Input: part model. Units: mm. Frame: model coordinates. A direction names the side the tool comes from. Give positions to 0.01 mm unless a question says otherwise; leave off trailing zeros. Loops run counter-clockwise (first coordinate to the right, second up) from the corner with the lowest first, then second, coordinate; pieces in that order, holes last. Notation, with made-up numbers: M -24,-20 L 9,-20 A35 ccw 9,14 Z; hole C 17.25,-9 d4. An arc over 180 degrees is marked long. Return JSON: item names as keys, results as strings. Group by question number.
```python
from build123d import *

# Parameters (mm, degrees)
EXTRUDE_1_DEPTH             = 20
HOLE_WIZARD_M41_D           = 4.5
HOLE_WIZARD_M41_DEPTH       = 5
HOLE_WIZARD_M41_TIP         = 1.351936393
HOLE_WIZARD_M21_D           = 1.6
HOLE_WIZARD_M21_DEPTH       = 6
HOLE_WIZARD_M21_CSINK_D     = 2.05
HOLE_WIZARD_M21_CSINK_ANGLE = 120
HOLE_WIZARD_M21_TIP         = 0.480688495


with BuildPart() as part:
    # Эскиз1 → Бобышка-Вытянуть1 (new body)
    with BuildSketch(Plane.XY):
        Polygon((0, 0), (0, 15), (2, 15), (2, 2), (15, 2), (15, 0), align=None)
    extrude(amount=EXTRUDE_1_DEPTH)

    # Отверстие с зазором M41
    with Locations(Plane(origin=(0, 2, 0), x_dir=(-1, 0, 0), z_dir=(0, 1, 0))):
        with Locations((-8, 5), (-8, 15)):
            Hole(HOLE_WIZARD_M41_D / 2, depth=HOLE_WIZARD_M41_DEPTH)
            with Locations((0, 0, -(HOLE_WIZARD_M41_DEPTH + HOLE_WIZARD_M41_TIP / 2))):  # 118° drill point
                Cone(0, HOLE_WIZARD_M41_D / 2, HOLE_WIZARD_M41_TIP, mode=Mode.SUBTRACT)

    # Отверстие обработанное метчиком M21
    with Locations(Plane(origin=(2, 0, 0), x_dir=(0, 0, -1), z_dir=(1, 0, 0))):
        with Locations((-4, 7), (-16, 7)):
            CounterSinkHole(HOLE_WIZARD_M21_D / 2, HOLE_WIZARD_M21_CSINK_D / 2, depth=HOLE_WIZARD_M21_DEPTH, counter_sink_angle=HOLE_WIZARD_M21_CSINK_ANGLE)
            with Locations((0, 0, -(HOLE_WIZARD_M21_DEPTH + HOLE_WIZARD_M21_TIP / 2))):  # 118° drill point
                Cone(0, HOLE_WIZARD_M21_D / 2, HOLE_WIZARD_M21_TIP, mode=Mode.SUBTRACT)


solid = part.part
```
Item 1: Pull-direction query (Y, two-part tool) for faces 1 (the face through (7.512, 0.986, 12.804)), 2 (the face through (0.92, 7.54, 15.41)), 3 (the face through (1, 15, 10)), 4 (the face through (0.92, 7.54, 3.41)); classes: pulls with the +Y half, pulls with the -Y half, needs draft (parallel to the pull), parting line crosses it, or undercut.
Item 2: First-contact query: pin 1 Ø7 at (x, z) = (8, 15) entering from +Y; pin 2 Ø1.8 at (y, z) = (7, 16) entering from +X; pin 3 Ø2 at (y, z) = (7, 4) entering from +X. Flat tips, straight axial feed; report the tip coordinate or a pass-through.
Item 3: Section C-C, the plane y = 4.5. Return loops of the section in (x, z), then the cut area to 3 significant figures.
Item 4: Material intervals for line 1 (Z direction, x = 0.5, y = 7); line 2 (Z direction, x = 8, y = 1.45); line 3 (Y direction, x = 0.7, z = 16), sorted ascending. Write a range as from..to.
Item 5: Section D-D, the plane z = 8.75. Return loops of the section in (x, y).
Item 6: Section B-B, the plane z = 4. Return loops of the section in (x, y) (3 decimals).
Item 7: Section A-A, the plane x = 8. Return loops of the section in (y, z).
Item 8: Reachability of faces 5 (the face through (8, 0, 10)), 6 (the face through (8, 2, 10)) from +Z, -Z, +X, -X, +Y, -Y: full face, straight path, thin tool, end or side. Return the list, or none.
Answer below:
{
 "1": {"face 1": "needs draft", "face 2": "undercut", "face 3": "pulls with the +Y half", "face 4": "undercut"},
 "2": {"pin 1": "y = 2", "pin 2": "x = 1.93", "pin 3": "x = 1.99"},
 "3": {"outline": "M 0,0 L 2,0 L 2,20 L 0,20 Z", "area": "40.0 mm^2"},
 "4": {"line 1": "0..3.2, 4.8..15.2, 16.8..20", "line 2": "0..2.75, 7.25..12.75, 17.25..20", "line 3": "0..6.2, 7.8..15"},
 "5": {"outline": "M 0,0 L 15,0 L 15,2 L 2,2 L 2,15 L 0,15 Z"},
 "6": {"outline": "M 0,0 L 5.984,0 L 5.984,2 L 2,2 L 2,5.975 L 1.87,6.2 L 0,6.2 Z; M 0,7.8 L 1.87,7.8 L 2,8.025 L 2,15 L 0,15 Z; M 10.016,0 L 15,0 L 15,2 L 10.016,2 Z"},
 "7": {"outline": "M 0,0 L 2,0 L 2,2.75 L 0,2.75 Z; M 0,7.25 L 2,7.25 L 2,12.75 L 0,12.75 Z; M 0,17.25 L 2,17.25 L 2,20 L 0,20 Z"},
 "8": {"face 5": "+Z, -Z, +X, -X, -Y", "face 6": "+Z, -Z, +X, +Y"}
}
